from build123d import *

# Parameters (mm, degrees)
SKETCH_R     = 16.5
PAD_DEPTH    = 6
SKETCH001_R  = 2
POCKET_DEPTH = 6.001
SKETCH002_R  = 2.5
PAD001_DEPTH = 2


with BuildPart() as part:
    # Sketch → Pad (new body)
    with BuildSketch(Plane.XY):
        Circle(SKETCH_R)
    extrude(amount=PAD_DEPTH)

    # Sketch001 (on Face3 of Pad) → Pocket (cut, through all)
    with BuildSketch(Plane.XY.offset(6)):
        with Locations((0, 16.5)):
            Circle(SKETCH001_R)
    extrude(amount=-POCKET_DEPTH, mode=Mode.SUBTRACT)

    # Sketch002 → Pad001 (join, symmetric)
    with BuildSketch(Plane.YZ):
        with BuildLine():
            Line((-10, 20), (-10, 0))
            Line((-10, 0), (10, 0))
            Line((10, 0), (10, 20))
            ThreePointArc((10, 20), (0, 30), (-10, 20))
        make_face()
        with Locations((0, 20)):
            Circle(SKETCH002_R, mode=Mode.SUBTRACT)
    extrude(amount=PAD001_DEPTH, both=True)


solid = part.part
Design review of the part built by this model. Coordinates are the model's own, in mm. A direction names the side the tool comes from. Round coordinates to 2 decimals unless told otherwise and drop trailing zeros. Write each loop counter-clockwise with the first axis right and the second up, starting at its lowest first coordinate (ties: lowest second). Pieces come first, ordered by that corner, then holes. Notation, with made-up numbers: (27.5, 9) - (63.5, 9) arc R16 cw to (63.5, 28) - close; hole circle Ø3 at (2.25, -5.75). An arc over 180 degrees is marked (long way). Use a Markdown table: item, result. Add a question column.
1. For faces 1 (the face through (0, 10, 13)), 2 (the face through (2, 0, 16)), 3 (the face through (0, -10, 13)), 4 (the face through (-0.697, -16.485, 2.958)), list the 3-axis set-ups (+Z, -Z, +X, -X, +Y, -Y) from which the entire face can be reached by the end or side of a thin tool; tool diameter is ignored.
2. We need section D-D (y = 7). State the section outline as (x, z) points.
3. We need section B-B (y = 0). State the section outline as (x, z) points, then the cut area to 3 significant figures.
4. We need section C-C (z = 2). State the section outline as (x, y) points, then the cut area to 3 significant figures.
5. Clearance check with flat-ended pins moving along their axes: pin 1 (3 mm diameter, centred on x = -0.5, z = 15, fed in from -Y); pin 2 (1.2 mm diameter, centred on x = 0, z = 13.5, fed in from +Y); pin 3 (3 mm diameter, centred on y = -6, z = 5, fed in from -X). State where each tip first meets the part, or that it passes through.
6. We need section A-A (x = 0). State the section outline as (y, z) points.
7. Mouldability with a two-part tool opening along Z and no side actions: class faces 5 (the face through (-2, 0, 16)), 6 (the face through (0, 0, 30)), 7 (the face through (0, 0, 0)), 8 (the face through (-0.03, -0.33, 22.48)) as +Z half, -Z half, draft (parallel to the pull), parting line (faces both ways), or undercut.
8. Wall thickness on probe 1 along Z at (x, y) = (-12.5, 9.5); probe 2 along Z at (x, y) = (0, 0); probe 3 along X at (y, z) = (6, 21.25): over which ranges is each line inside the solid? List them lowest first.
Output:
| question | item | result |
|---|---|---|
| 1 | face 1 | +Z, +X, -X, +Y |
| 1 | face 2 | +Z, +X, +Y, -Y |
| 1 | face 3 | +Z, +X, -X, -Y |
| 1 | face 4 | +Z, -Z |
| 2 | outline | (-14.94, 0) - (14.94, 0) - (14.94, 6) - (2, 6) - (2, 27.14) - (-2, 27.14) - (-2, 6) - (-14.94, 6) - close |
| 3 | outline | (-16.5, 0) - (16.5, 0) - (16.5, 6) - (2, 6) - (2, 17.5) - (-2, 17.5) - (-2, 6) - (-16.5, 6) - close; (-2, 22.5) - (2, 22.5) - (2, 30) - (-2, 30) - close |
| 3 | area | 274 mm2 |
| 4 | outline | (-2, 16.38) arc R16.5 ccw (long way) to (2, 16.38) arc R2 cw to start |
| 4 | area | 849 mm2 |
| 5 | pin 1 | stops at y = -10 |
| 5 | pin 2 | stops at y = 10 |
| 5 | pin 3 | stops at x = -15.87 |
| 6 | outline | (-16.5, 0) - (14.5, 0) - (14.5, 6) - (10, 6) - (10, 20) arc R10 ccw to (-10, 20) - (-10, 6) - (-16.5, 6) - close; hole circle Ø5 at (0, 20) |
| 7 | face 5 | draft |
| 7 | face 6 | +Z half |
| 7 | face 7 | -Z half |
| 7 | face 8 | undercut |
| 8 | probe 1 | z = 0 to 6 |
| 8 | probe 2 | z = 0 to 17.5, 22.5 to 30 |
| 8 | probe 3 | x = -2 to 2 |
